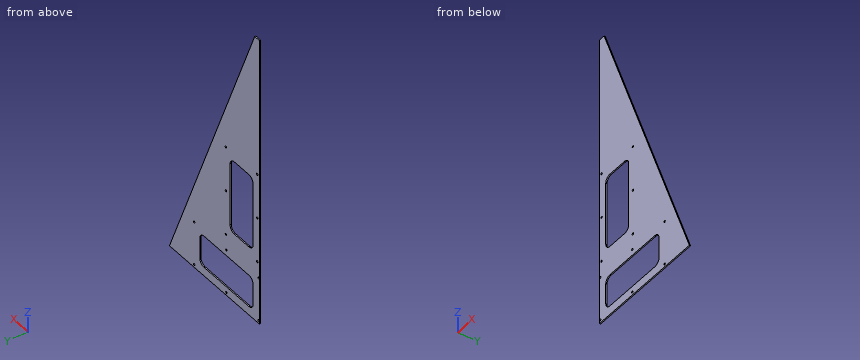
```python
from build123d import *

# Parameters (mm, degrees)
F1_DEPTH = 2.54
F3_D     = 4.318


with BuildPart() as f1:
    # F0 (on Front) → F1 (new body)
    with BuildSketch(Plane.XZ):
        Polygon((0, 635), (0, 0), (273.05, 0), (14.0198087095, 635), align=None)
        with BuildLine():
            Line((168.275, 19.05), (31.75, 19.05))
            ThreePointArc((31.75, 19.05), (22.7697438789, 22.7697438789), (19.05, 31.75))
            Line((19.05, 31.75), (19.05, 76.2))
            ThreePointArc((19.05, 76.2), (22.7697438789, 85.1802561211), (31.75, 88.9))
            Line((31.75, 88.9), (168.275, 88.9))
            ThreePointArc((168.275, 88.9), (177.2552561211, 85.1802561211), (180.975, 76.2))
            Line((180.975, 76.2), (180.975, 31.75))
            ThreePointArc((180.975, 31.75), (177.2552561211, 22.7697438789), (168.275, 19.05))
        make_face(mode=Mode.SUBTRACT)
        with BuildLine():
            Line((76.2, 152.4), (31.75, 152.4))
            ThreePointArc((31.75, 152.4), (22.7697438789, 156.1197438789), (19.05, 165.1))
            Line((19.05, 165.1), (19.05, 301.625))
            ThreePointArc((19.05, 301.625), (22.7697438789, 310.6052561211), (31.75, 314.325))
            Line((31.75, 314.325), (76.2, 314.325))
            ThreePointArc((76.2, 314.325), (85.1802561211, 310.6052561211), (88.9, 301.625))
            Line((88.9, 301.625), (88.9, 165.1))
            ThreePointArc((88.9, 165.1), (85.1802561211, 156.1197438789), (76.2, 152.4))
        make_face(mode=Mode.SUBTRACT)
    extrude(amount=F1_DEPTH)

    # F3 (through all)
    with Locations(Plane.XZ.offset(2.54)):
        with Locations((6.35, 331.1525), (101.6, 331.1525), (101.6, 233.3625), (6.35, 233.3625), (6.35, 135.5725), (101.6, 135.5725), (2.2225, 101.6), (2.2225, 6.35), (100.0125, 6.35), (100.0125, 101.6), (197.8025, 101.6), (197.8025, 6.35)):
            Hole(F3_D / 2)


solid = f1.part
```
Input: part model. Units: mm. Frame: model coordinates. Give positions to 0.01 mm unless a question says otherwise; leave off trailing zeros. Order: outer loops, then holes, each group sorted by start corner. A loop starts at its lowest first (then second) coordinate and runs counter-clockwise, first axis right, second up. Notation, with made-up numbers: M 33.5,55 L 58.5,55 A12 cw 58.5,62 Z; hole C -31.5,-34.75 d8. An arc over 180 degrees is marked long. One line per question, with ' | ' between items. Start each with the question number.
1. Material intervals for probe 1 along Z at (x, y) = (6.35, -0.55); probe 2 along Z at (x, y) = (52, -1.6) (3 decimals); probe 3 along Z at (x, y) = (157, -1.6), sorted ascending. Write a range as [from, to].
2. Section query A-A (z = 210). Return the cut outline in (x, y), and give its area (3 significant figures).
3. Section query B-B (y = -1.55). Count the separate pieces of the cut face and the enclosed holes in it, and give its area (3 significant figures).
4. First-contact query: pin 1 Ø1 at (x, z) = (172, 135.5) entering from +Y; pin 2 Ø0.8 at (x, y) = (114, -1) entering from +Z; pin 3 Ø1.3 at (y, z) = (-1.5, 65) entering from +X; pin 4 Ø0.8 at (y, z) = (-1, 235) entering from +X. Flat tips, straight axial feed; report the tip coordinate or a pass-through.
5. Section query D-D (z = 459). Return the cut outline in (x, y), and give its area (3 significant figures).
6. Section query C-C (x = 129). Return the cut outline in (y, z).
Here are the results:
1) probe 1: [0, 133.41], [137.73, 231.2], [235.52, 328.99], [333.31, 635] | probe 2: [0, 19.05], [88.9, 152.4], [314.325, 541.893] | probe 3: [0, 19.05], [88.9, 284.49]
2) outline: M 0,-2.54 L 19.05,-2.54 L 19.05,0 L 0,0 Z; M 88.9,-2.54 L 187.39,-2.54 L 187.39,0 L 88.9,0 Z | area: 299 mm²
3) separate pieces: 1 | enclosed holes: 14 | area: 68,600 mm²
4) pin 1: y = 0 | pin 2: z = 390.88 | pin 3: x = 246.8 | pin 4: x = 177.35
5) outline: M 0,-2.54 L 85.81,-2.54 L 85.81,0 L 0,0 Z | area: 218 mm²
6) outline: M -2.54,0 L 0,0 L 0,19.05 L -2.54,19.05 Z; M -2.54,88.9 L 0,88.9 L 0,353.13 L -2.54,353.13 Z
